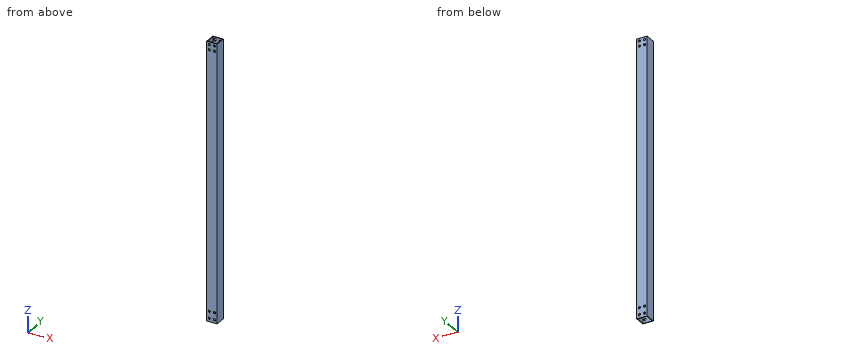
from build123d import *

# Parameters (mm, degrees)
SKETCH_1_W          = 15
SKETCH_1_H          = 15
SKETCH_1_W_2        = 13
SKETCH_1_H_2        = 13
EXTRUDE_1_DEPTH     = 400
SKETCH_2_R          = 1.6
CUT_EXTRUDE_1_DEPTH = 401.562105047


with BuildPart() as part:
    # 草图1 → 拉伸-薄壁1 (new body)
    with BuildSketch(Plane.XY):
        with Locations((7.5, -7.5)):
            Rectangle(SKETCH_1_W, SKETCH_1_H)
        with Locations((7.5, -7.5)):
            Rectangle(SKETCH_1_W_2, SKETCH_1_H_2, mode=Mode.SUBTRACT)
    extrude(amount=EXTRUDE_1_DEPTH)

    # 草图2 → 切除-拉伸1 (cut, through all)
    with BuildSketch(Plane(origin=(0, 0, 0), x_dir=(1, 0, 0), z_dir=(0, 1, 0))):
        with Locations(Location((3.75, -5, 0), (0, 0, 270))):
            Circle(SKETCH_2_R)
        with Locations(Location((11.25, -5, 0), (0, 0, 90))):
            Circle(SKETCH_2_R)
        with Locations(Location((11.25, -15, 0), (0, 0, 270))):
            Circle(SKETCH_2_R)
        with Locations(Location((3.75, -15, 0), (0, 0, 90))):
            Circle(SKETCH_2_R)
        with Locations(Location((3.75, -396.25, 0), (0, 0, 270))):
            Circle(SKETCH_2_R)
        with Locations(Location((11.25, -396.25, 0), (0, 0, 90))):
            Circle(SKETCH_2_R)
        with Locations(Location((11.25, -388.75, 0), (0, 0, 270))):
            Circle(SKETCH_2_R)
        with Locations(Location((3.75, -388.75, 0), (0, 0, 90))):
            Circle(SKETCH_2_R)
    extrude(amount=-CUT_EXTRUDE_1_DEPTH, mode=Mode.SUBTRACT)


solid = part.part
Work out the finished part from the listing and answer in its coordinate system (mm). Give positions to 0.01 mm unless a question says otherwise; leave off trailing zeros. Loops run counter-clockwise (first coordinate to the right, second up) from the corner with the lowest first, then second, coordinate; pieces in that order, holes last. Notation, with made-up numbers: (19, 15) - (48, 15) arc R23 ccw to (48, 41) - close; hole circle Ø10 at (84.25, -3). An arc over 180 degrees is marked (long way). Answer in a Markdown table with one row per item.
(1) Section B-B (z = 356) is taken. Give the vertices of the cut face in (x, y), and give its area (3 significant figures).
Results list:
| item | result |
|---|---|
| outline | (0, -15) - (15, -15) - (15, 0) - (0, 0) - close; hole (1, -14) - (14, -14) - (14, -1) - (1, -1) - close |
| area | 56.0 mm² |
(2) Consider L1, parallel to X at y = -0.3, z = 388.75; L2, parallel to Y at x = 6.25, z = 250; L3, parallel to X at y = -10.25, z = 212.5. Determine where each line is inside the solid, lowest interval first. Write a range as [from, to].
Results list:
| item | result |
|---|---|
| L1 | x = [0, 2.15], [5.35, 9.65], [12.85, 15] |
| L2 | y = [-15, -14], [-1, 0] |
| L3 | x = [0, 1], [14, 15] |
(3) Section A-A (y = -7) is taken. Give the vertices of the cut face in (x, z), and give its area (3 significant figures).
Results list:
| item | result |
|---|---|
| outline | (0, 0) - (1, 0) - (1, 400) - (0, 400) - close; (14, 0) - (15, 0) - (15, 400) - (14, 400) - close |
| area | 800 mm² |
